```python
from build123d import *

# Parameters (mm, degrees)
F0_W      = 23
F0_H      = 12.5
F1_DEPTH  = 23
F3_W      = 33
F3_H      = 12.5
F4_DEPTH  = 3
F6_DEPTH  = 5.5
F7_R      = 2.4
F8_DEPTH  = 4
F10_DEPTH = 25


with BuildPart() as f1:
    # F0 (on Top) → F1 (new body)
    with BuildSketch(Plane.XY):
        with Locations((-21.4128988087, -13.7193646282)):
            Rectangle(F0_W, F0_H)
    extrude(amount=F1_DEPTH)

    # F3 (on offset) → F4 (join)
    with BuildSketch(Plane.XY.offset(21.7)):
        with Locations((-21.4128988087, -13.7193646282)):
            Rectangle(F3_W, F3_H)
    extrude(amount=-F4_DEPTH)

    # F5 (on face) → F6 (join)
    with BuildSketch(Plane.XY.offset(23)):
        with BuildLine():
            ThreePointArc((-26.6628988087, -19.9693646282), (-22.2434814263, -18.1387820106), (-20.4128988087, -13.7193646282))
            ThreePointArc((-20.4128988087, -13.7193646282), (-22.2434814263, -9.2999472458), (-26.6628988087, -7.4693646282))
            ThreePointArc((-26.6628988087, -7.4693646282), (-31.0823161911, -9.2999472458), (-32.9128988087, -13.7193646282))
            ThreePointArc((-32.9128988087, -13.7193646282), (-31.0823161911, -18.1387820106), (-26.6628988087, -19.9693646282))
        make_face()
    extrude(amount=F6_DEPTH)

    # F7 (on face) → F8 (join)
    with BuildSketch(Plane.XY.offset(28.5)):
        with Locations((-26.6628988087, -13.7193646282)):
            Circle(F7_R)
    extrude(amount=F8_DEPTH)

    # F9 (on face) → F10 (cut)
    with BuildSketch(Plane.XY.offset(21.7)):
        with BuildLine():
            ThreePointArc((-37.8123308197, -14.2869679257), (-36.5777129376, -14.9020368395), (-35.7128988087, -13.8274729252))
            ThreePointArc((-35.7128988087, -13.8274729252), (-36.5409103144, -12.7616294756), (-37.778393825, -13.3003871888))
            Line((-37.778393825, -13.3003871888), (-37.1418111026, -13.3003871888))
            Line((-37.1418111026, -13.3003871888), (-37.1418111026, -13.7193646282))
            Line((-37.1418111026, -13.7193646282), (-37.1418111026, -14.2869679257))
            Line((-37.1418111026, -14.2869679257), (-37.8123308197, -14.2869679257))
        make_face()
        with BuildLine():
            Line((-37.1418111026, -13.3003871888), (-37.778393825, -13.3003871888))
            ThreePointArc((-37.778393825, -13.3003871888), (-37.8640697227, -13.5033746227), (-37.9075734618, -13.7193646282))
            Line((-37.9075734618, -13.7193646282), (-37.1418111026, -13.7193646282))
            Line((-37.1418111026, -13.7193646282), (-37.1418111026, -13.3003871888))
        make_face()
        with BuildLine():
            ThreePointArc((-37.9075734618, -13.7193646282), (-37.8640697227, -13.5033746227), (-37.778393825, -13.3003871888))
            Line((-37.778393825, -13.3003871888), (-38.5551899672, -13.3003871888))
            Line((-38.5551899672, -13.3003871888), (-38.5551899672, -13.7193646282))
            Line((-38.5551899672, -13.7193646282), (-37.9075734618, -13.7193646282))
        make_face()
        with BuildLine():
            Line((-38.5551899672, -14.2869679257), (-37.8123308197, -14.2869679257))
            ThreePointArc((-37.8123308197, -14.2869679257), (-37.8977324623, -14.0095057356), (-37.9075734618, -13.7193646282))
            Line((-37.9075734618, -13.7193646282), (-38.5551899672, -13.7193646282))
            Line((-38.5551899672, -13.7193646282), (-38.5551899672, -14.2869679257))
        make_face()
        with BuildLine():
            ThreePointArc((-37.9075734618, -13.7193646282), (-37.8977324623, -14.0095057356), (-37.8123308197, -14.2869679257))
            Line((-37.8123308197, -14.2869679257), (-37.1418111026, -14.2869679257))
            Line((-37.1418111026, -14.2869679257), (-37.1418111026, -13.7193646282))
            Line((-37.1418111026, -13.7193646282), (-37.9075734618, -13.7193646282))
        make_face()
    extrude(amount=-F10_DEPTH, mode=Mode.SUBTRACT)


solid = f1.part
```
Geometry: final body of the model. Coordinates: model frame, mm. A direction names the side the tool comes from. Coordinates: 2 decimals unless noted, no trailing zeros. Loops run counter-clockwise (first coordinate to the right, second up) from the corner with the lowest first, then second, coordinate; pieces in that order, holes last. Notation, with made-up numbers: (-8, 84) -> (39, 84) arc R10 ccw to (39, 90) -> close; hole circle Ø2 at (-30, 76). An arc over 180 degrees is marked (long way). Use a Markdown table: item, result. Add a question column.
(1) Section query B-B, the plane x = -14.5. Return loops of the section in (y, z), plus the area to 4 significant figures.
(2) Pin query (flat end, axial travel): pin 1 Ø5.5 at (x, y) = (-36.5, -12.5) entering from -Z; pin 2 Ø2.5 at (x, y) = (-8.5, -15.5) entering from +Z; pin 3 Ø6 at (x, y) = (-8.5, -14.5) entering from +Z. Return the tip coordinate at first contact, or that it passes through.
(3) Access query for faces 1 (the flat face through (-7, -14, 18.7)), 2 (the cylindrical face through (-29.06, -13.61, 30.47)), 3 (the flat face through (-35, -14, 21.7)). Directions: +Z, -Z, +X, -X, +Y, -Y. A direction counts if a zero-diameter tool reaches every point of the face in a straight line with its end or side. Return the directions, or none.
(4) Section query D-D, the plane y = -11.75. Return loops of the section in (x, z), plus the area to 3 significant figures.
(5) Line query: line 1 along Z through (x, y) = (-20.5, -10); line 2 along X through (y, z) = (-16.5, 15); line 3 along Z through (x, y) = (-28.5, -16.75). Output: solid intervals per line, ascending.
(6) Section query A-A, the plane y = -9. Return loops of the section in (x, z).
(7) Section query C-C, the plane z = 29. Return loops of the section in (x, y).
Answer:
| question | item | result |
|---|---|---|
| 1 | outline | (-19.97, 0) -> (-7.47, 0) -> (-7.47, 23) -> (-19.97, 23) -> close |
| 1 | area | 287.5 mm^2 |
| 2 | pin 1 | stops at z = 18.7 |
| 2 | pin 2 | stops at z = 21.7 |
| 2 | pin 3 | stops at z = 23 |
| 3 | face 1 | -Z, +X, +Y, -Y |
| 3 | face 2 | +Z |
| 3 | face 3 | +Z, -X, +Y, -Y |
| 4 | outline | (-37.91, 18.7) -> (-32.91, 18.7) -> (-32.91, 0) -> (-9.91, 0) -> (-9.91, 18.7) -> (-4.91, 18.7) -> (-4.91, 21.7) -> (-9.91, 21.7) -> (-9.91, 23) -> (-20.73, 23) -> (-20.73, 28.5) -> (-25.29, 28.5) -> (-25.29, 32.5) -> (-28.03, 32.5) -> (-28.03, 28.5) -> (-32.59, 28.5) -> (-32.59, 23) -> (-32.91, 23) -> (-32.91, 21.7) -> (-37.91, 21.7) -> close |
| 4 | area | 635 mm^2 |
| 5 | line 1 | z = 0 to 23 |
| 5 | line 2 | x = -32.91 to -9.91 |
| 5 | line 3 | z = 0 to 28.5 |
| 6 | outline | (-37.91, 18.7) -> (-32.91, 18.7) -> (-32.91, 0) -> (-9.91, 0) -> (-9.91, 18.7) -> (-4.91, 18.7) -> (-4.91, 21.7) -> (-9.91, 21.7) -> (-9.91, 23) -> (-22.57, 23) -> (-22.57, 28.5) -> (-30.76, 28.5) -> (-30.76, 23) -> (-32.91, 23) -> (-32.91, 21.7) -> (-37.91, 21.7) -> close |
| 7 | outline | circle Ø4.8 at (-26.66, -13.72) |
